```python
from build123d import *

# Parameters (mm, degrees)
BOSS_EXTRU_1_DEPTH           = 35
COQUE1_START                 = 4
COQUE1_DEPTH                 = 31
ESQUISSE2_R                  = 1.5
BOSS_EXTRU_2_DEPTH           = 4
ENL_V_MAT_EXTRU_1_DEPTH      = 175.132380731
ENL_V_MAT_EXTRU_1_DEPTH_BACK = 175.132380731
ESQUISSE3_R                  = 2
ENL_V_MAT_EXTRU_3_REACH      = 176.132


# Read off the part's stored shape, not the designer's step: Coque1
with BuildPart() as part:
    # Esquisse1 → Boss.-Extru.1 (new body)
    with BuildSketch(Plane.XY):
        with BuildLine():
            Line((0, 0), (32, 0))
            ThreePointArc((32, 0), (55.728066531, 42.841616018), (42.820629182, 90.083792782))
            ThreePointArc((42.820629182, 90.083792782), (33.698409335, 113.699589876), (41.435424367, 137.804762884))
            ThreePointArc((41.435424367, 137.804762884), (25.22744291, 121.551637289), (19.984387859, 99.204979189))
            ThreePointArc((19.984387859, 99.204979189), (12.61609693, 111.881969553), (12.136039681, 126.536912097))
            ThreePointArc((12.136039681, 126.536912097), (4.219515773, 112.802914106), (2.969732835, 97))
            ThreePointArc((2.969732835, 97), (-3.409170119, 104.566084027), (-6.3525056, 114.014512821))
            ThreePointArc((-6.3525056, 114.014512821), (-10.072723061, 102.291129965), (-8.812437557, 90.056367852))
            ThreePointArc((-8.812437557, 90.056367852), (-5.254890234, 75.901823785), (-8.797583956, 61.743554757))
            ThreePointArc((-8.797583956, 61.743554757), (-17.657714331, 28.982568326), (0, 0))
        make_face()
    extrude(amount=BOSS_EXTRU_1_DEPTH)

    # Coque1 outline → Coque1 (cut)
    with BuildSketch(Plane.XY.offset(COQUE1_START)):
        with BuildLine():
            ThreePointArc((-5.450317373, 59.524921192), (-13.80168075, 30.333767047), (1.311276064, 4))
            Line((1.311276064, 4), (30.562561826, 4))
            ThreePointArc((30.562561826, 4), (51.829960407, 43.957714999), (39.70782155, 87.569353124))
            ThreePointArc((39.70782155, 87.569353124), (31.129906971, 103.87080592), (30.352555686, 122.274982261))
            ThreePointArc((30.352555686, 122.274982261), (24.349701453, 106.719246419), (25.584028276, 90.091209439))
            ThreePointArc((25.584028276, 90.091209439), (14.515213943, 99.414058708), (8.326368872, 112.495815697))
            ThreePointArc((8.326368872, 112.495815697), (6.635364168, 100.670475038), (9.39901844, 89.048926361))
            ThreePointArc((9.39901844, 89.048926361), (0.546946732, 93.816298878), (-6.145312397, 101.319676916))
            ThreePointArc((-6.145312397, 101.319676916), (-6.081248931, 96.409310993), (-5.102512487, 91.597048261))
            ThreePointArc((-5.102512487, 91.597048261), (-1.256885168, 75.517395098), (-5.450317373, 59.524921192))
        make_face()
    extrude(amount=COQUE1_DEPTH, mode=Mode.SUBTRACT)

    # Esquisse2 → Boss.-Extru.2 (add)
    # profile 1 of 2: a face of its own
    with BuildSketch(Plane.XY):
        with BuildLine():
            Line((32, 0), (32, 12.299667719))
            ThreePointArc((32, 12.299667719), (58.802567763, 44.999332283), (63.659481669, 87))
            ThreePointArc((63.659481669, 87), (75.517173587, 52.886347991), (63.659481669, 18.772695982))
            ThreePointArc((63.659481669, 18.772695982), (83.222118055, 26.227396664), (100.533244977, 38))
            ThreePointArc((100.533244977, 38), (73.327044482, 6.266483418), (32, 0))
        make_face()
        with Locations((69.376907093, 65)):
            Circle(ESQUISSE2_R, mode=Mode.SUBTRACT)
        with Locations((82, 20)):
            Circle(ESQUISSE2_R, mode=Mode.SUBTRACT)
    # profile 2 of 2: a face of its own
    with BuildSketch(Plane.XY):
        with BuildLine():
            Line((0, 0), (0, 12.299667719))
            ThreePointArc((0, 12.299667719), (-26.802567763, 44.999332283), (-31.659481669, 87))
            ThreePointArc((-31.659481669, 87), (-43.517173587, 52.886347991), (-31.659481669, 18.772695982))
            ThreePointArc((-31.659481669, 18.772695982), (-51.222118055, 26.227396664), (-68.533244977, 38))
            ThreePointArc((-68.533244977, 38), (-41.327044482, 6.266483418), (0, 0))
        make_face()
        with Locations(Location((-50, 20, 0), (0, 0, 180))):
            Circle(ESQUISSE2_R, mode=Mode.SUBTRACT)
        with Locations(Location((-37.376907093, 65, 0), (0, 0, 180))):
            Circle(ESQUISSE2_R, mode=Mode.SUBTRACT)
    extrude(amount=BOSS_EXTRU_2_DEPTH)

    # Esquisse3 → Enlèv. mat.-Extru.1 (cut, two sides: drawn at the far end of the back side and taken through both)
    with BuildSketch(Plane(origin=(0, 0, 0), x_dir=(0, 0, -1), z_dir=(1, 0, 0)).offset(-ENL_V_MAT_EXTRU_1_DEPTH_BACK)):
        with Locations((-20, 55)):
            Circle(ESQUISSE3_R)
    extrude(amount=ENL_V_MAT_EXTRU_1_DEPTH + ENL_V_MAT_EXTRU_1_DEPTH_BACK, mode=Mode.SUBTRACT)

    # Esquisse4 → Enlèv. mat.-Extru.3 (cut, up to next)
    with BuildSketch(Plane.XZ, mode=Mode.PRIVATE) as enl_v_mat_extru_3_sk1:
        with BuildLine():
            Line((13.536266916, 16), (18.463733084, 16))
            ThreePointArc((18.463733084, 16), (18.499418045, 16.00320929), (18.533957772, 16.012734164))
            Line((18.533957772, 16.012734164), (20.370224688, 16.701334258))
            ThreePointArc((20.370224688, 16.701334258), (20.464385124, 16.774681126), (20.5, 16.888600094))
            Line((20.5, 16.888600094), (20.5, 17.3))
            ThreePointArc((20.5, 17.3), (20.441421356, 17.441421356), (20.3, 17.5))
            Line((20.3, 17.5), (11.7, 17.5))
            ThreePointArc((11.7, 17.5), (11.558578644, 17.441421356), (11.5, 17.3))
            Line((11.5, 17.3), (11.5, 16.888600094))
            ThreePointArc((11.5, 16.888600094), (11.535614876, 16.774681126), (11.629775312, 16.701334258))
            Line((11.629775312, 16.701334258), (13.536266916, 16))
        make_face()
    enl_v_mat_extru_3_tool1 = extrude(enl_v_mat_extru_3_sk1.sketch, amount=-ENL_V_MAT_EXTRU_3_REACH, mode=Mode.PRIVATE) & part.part
    add(enl_v_mat_extru_3_tool1.solids().sort_by_distance((16.003291, 0, 16.812223))[0], mode=Mode.SUBTRACT)


solid = part.part
```
CAD build for the part. Positions are in the model's coordinates, mm. A direction names the side the tool comes from. Coordinates: 2 decimals unless noted, no trailing zeros. Write each loop counter-clockwise with the first axis right and the second up, starting at its lowest first coordinate (ties: lowest second). Pieces come first, ordered by that corner, then holes. Notation, with made-up numbers: (6, -22.75) -> (36, -22.75) arc R15 ccw to (36, -17.75) -> close; hole circle Ø2 at (-17.5, 5). An arc over 180 degrees is marked (long way). Return JSON: item names as keys, results as strings. Group by question number.
Q1. Cut at A-A, the plane z = 27.5. Give the cut face in (x, y), then the cut area to 3 significant figures.
Q2. Cut at C-C, the plane x = 48. Give the cut face in (y, z).
Q3. Flat gauge pins, fed straight in: pin 1 (6 mm diameter, centred on x = 36.5, z = 7, fed in from +Y); pin 2 (5 mm diameter, centred on y = 46, z = 20.5, fed in from +X); pin 3 (4 mm diameter, centred on y = 15.5, z = 26.5, fed in from -X); pin 4 (2.5 mm diameter, centred on x = -50, y = 20, fed in from +Z). Where does each tip first touch, or does it go through?
Q4. Pull direction X, two halves, no side cores. Call faces 1 (the face through (15, 54, 0)), 2 (the face through (-10.055, 102.464, 17.255)), 3 (the face through (75.515, 53.402, 1.972)): released by +X, released by -X, zero draft, split by the parting line, or undercut.
Q5. Cut at B-B, the plane y = 35. Give the cut face in (x, z), then the cut area to 3 significant figures.
Q6. Drill centre lines: line 1 (Y direction, x = -50, z = 2); line 2 (X direction, y = 91.5, z = 24); line 3 (X direction, y = 102.5, z = 27). Where is each one in solid material? Low to high.
Q7. Which spindle directions (+Z, -Z, +X, -X, +Y, -Y) get a long thin tool onto all of the face, cutting with end or side? Do faces 4 (the face through (16, 2, 17.5)), 5 (the face through (-34, 27, 4)), 6 (the face through (-13.852, 30.767, 19.283)), 7 (the face through (64, 30, 4)). Say none if no direction does.
Returned:
{
 "1": {"outline": "(-8.81, 90.06) arc R30 cw to (-8.8, 61.74) arc R43 ccw to (0, 0) -> (32, 0) arc R65 ccw to (42.82, 90.08) arc R38 cw to (41.44, 137.8) arc R42 ccw to (19.98, 99.2) arc R30 cw to (12.14, 126.54) arc R36 ccw to (2.97, 97) arc R25 cw to (-6.35, 114.01) arc R30.22 ccw to start; hole (-6.15, 101.32) arc R26.22 ccw to (-5.1, 91.6) arc R34 cw to (-5.45, 59.52) arc R39 ccw to (1.31, 4) -> (30.56, 4) arc R61 ccw to (39.71, 87.57) arc R42 cw to (30.35, 122.27) arc R38 ccw to (25.58, 90.09) arc R34 cw to (8.33, 112.5) arc R32 ccw to (9.4, 89.05) arc R29 cw to start", "area": "1,620 mm2"},
 "2": {"outline": "(-1.14, 0) -> (82.18, 0) -> (82.18, 35) -> (72.82, 35) -> (72.82, 4) -> (28.37, 4) -> (28.37, 35) -> (19, 35) -> (19, 4) -> (-1.14, 4) -> close"},
 "3": {"pin 1": "stops at y = 136.65", "pin 2": "stops at x = 56.16", "pin 3": "stops at x = -14.34", "pin 4": "passes through"},
 "4": {"face 1": "zero draft", "face 2": "released by -X", "face 3": "undercut"},
 "5": {"outline": "(-67.34, 0) -> (-64.88, 0) -> (-64.88, 4) -> (-67.34, 4) -> close; (-40.53, 0) -> (-21.65, 0) -> (-21.65, 4) -> (-40.53, 4) -> close; (-18.09, 0) -> (72.53, 0) -> (72.53, 4) -> (54.29, 4) -> (54.29, 35) -> (50.17, 35) -> (50.17, 4) -> (-14.09, 4) -> (-14.09, 35) -> (-18.09, 35) -> close; (96.88, 0) -> (99.34, 0) -> (99.34, 4) -> (96.88, 4) -> close", "area": "710 mm2"},
 "6": {"line 1": "y = 12.12 to 18.5, 21.5 to 25.6", "line 2": "x = -9.23 to -5.05, 3.95 to 8.42, 23.16 to 25.18, 36.74 to 41.67", "line 3": "x = -10.05 to -2.14, 2.6 to 6.6, 12.4 to 17.2, 19.96 to 23.96, 31.52 to 35.73"},
 "7": {"face 4": "-Y", "face 5": "+Z, -X, -Y", "face 6": "+Z", "face 7": "+Z, +X, -Y"}
}
